For this review, take the finished solid that the model builds, in its own axes (mm). A direction names the side the tool comes from. Coordinates: 2 decimals unless noted, no trailing zeros. Order: outer loops, then holes, each group sorted by start corner. A loop starts at its lowest first (then second) coordinate and runs counter-clockwise, first axis right, second up.
from build123d import *

# Parameters (mm, degrees)
CROQUIS1_W              = 45
CROQUIS1_H              = 70
SALIENTE_EXTRUIR1_DEPTH = 2
CROQUIS2_W              = 23
CROQUIS2_H              = 3.3
CORTAR_EXTRUIR1_DEPTH   = 2
REDONDEO1_R             = 3
REDONDEO2_R             = 0.5


with BuildPart() as part:
    # Croquis1 → Saliente-Extruir1 (new body)
    with BuildSketch(Plane(origin=(0, 0, 0), x_dir=(1, 0, 0), z_dir=(0, 1, 0))):
        with Locations((0, 0.306231574)):
            Rectangle(CROQUIS1_W, CROQUIS1_H)
    extrude(amount=SALIENTE_EXTRUIR1_DEPTH)

    # Croquis2 → Cortar-Extruir1 (cut)
    with BuildSketch(Plane(origin=(0, 2, 0), x_dir=(1, 0, 0), z_dir=(0, 1, 0))):
        with Locations((-11, -29.35)):
            Rectangle(CROQUIS2_W, CROQUIS2_H)
    extrude(amount=-CORTAR_EXTRUIR1_DEPTH, mode=Mode.SUBTRACT)

    # Redondeo1
    redondeo1_edges = [part.edges().sort_by_distance(p)[0] for p in [
        (-22.5, 1, -35.306231574),
        (22.5, 1, -35.306231574),
        (22.5, 1, 34.693768426),
        (-22.5, 1, 34.693768426),
    ]]
    fillet(redondeo1_edges, radius=REDONDEO1_R)

    # Redondeo2
    redondeo2_edges = [part.edges().sort_by_distance(p)[0] for p in [
        (-22.5, 1, 31),
        (-22.5, 1, 27.7),
        (0.5, 1, 27.7),
        (0.5, 1, 31),
    ]]
    fillet(redondeo2_edges, radius=REDONDEO2_R)


solid = part.part
1. Take a section at A-A, the plane x = -8. Give the boundary of the cut face in (y, z).
Answer below:
outline: (0, -35.31) - (2, -35.31) - (2, 27.7) - (0, 27.7) - close; (0, 31) - (2, 31) - (2, 34.69) - (0, 34.69) - close
2. Machinability: for faces 4 (the face through (-21.645, 1.014, 33.792)), 5 (the face through (0.5, 1, 29)), which of the approach directions +Z, -Z, +X, -X, +Y, -Y give a long, thin tool a straight path to every point of the face, cutting with its end or side? Answer none if there is none.
Answer below:
face 4: +Z, -X, +Y, -Y
face 5: -X, +Y, -Y
3. To check wall thickness, follow L1, parallel to Z at x = -14.5, y = 1.7. State the ranges of the line that lie inside material, in increasing order.
Answer below:
L1: z = -35.31 to 27.7, 31 to 34.69
4. The part is to be moulded in two halves that separate along Z. For faces 1 (the face through (0, 0, -1)), 2 (the face through (-21.645, 1.014, -34.404)), 3 (the face through (-11, 1, 27.7)), say which applies: +Z half, -Z half, draft (parallel to the pull), parting line (faces both ways), or undercut.
Answer below:
face 1: draft
face 2: -Z half
face 3: undercut
5. Take a section at B-B, the plane y = 0.9. Give the boundary of the cut face in (x, z).
Answer below:
outline: (-22.5, -32.31) arc R3 ccw to (-19.5, -35.31) - (19.5, -35.31) arc R3 ccw to (22.5, -32.31) - (22.5, 31.69) arc R3 ccw to (19.5, 34.69) - (-19.5, 34.69) arc R3 ccw to (-22.5, 31.69) - (-22.5, 31.5) arc R0.5 ccw to (-22, 31) - (0, 31) arc R0.5 cw to (0.5, 30.5) - (0.5, 28.2) arc R0.5 cw to (0, 27.7) - (-22, 27.7) arc R0.5 ccw to (-22.5, 27.2) - close
6. Take a section at C-C, the plane z = 29. Give the boundary of the cut face in (x, y).
Answer below:
outline: (0.5, 0) - (22.5, 0) - (22.5, 2) - (0.5, 2) - close
